Read the model definition and answer for the solid it produces. Units are mm, in the model's axes. Face numbers are marked on the shaded views. Coordinates: 2 decimals unless noted, no trailing zeros. Write each loop counter-clockwise with the first axis right and the second up, starting at its lowest first coordinate (ties: lowest second). Pieces come first, ordered by that corner, then holes.
1) The part is cut by section B-B (y = 0). Determine the outline of the cut face in (x, z).
2) The part is cut by section A-A (x = -6.35). Determine the outline of the cut face in (y, z), then the cut area to 3 significant figures.
3) Find the intervals of material crossed by line 1 (Y direction, x = -4, z = 19); line 2 (Z direction, x = -3.5, y = 1); line 3 (Y direction, x = -6, z = 26), in increasing order.
4) Determine the mould class of the marked faces 1, 2, 3 and 4 for opening direction Y: +Y half, -Y half, draft (parallel to the pull), parting line (faces both ways), or undercut.
5) Each of these flat-tipped pins is pushed along its axis until it touches: pin 1 Ø6 at (y, z) = (-4.5, -7.5) entering from -X; pin 2 Ø12 at (x, z) = (-16, -2) entering from -Y; pin 3 Ø7.5 at (x, y) = (-6.5, 0) entering from +Z. Where does it stop, or does it pass through?
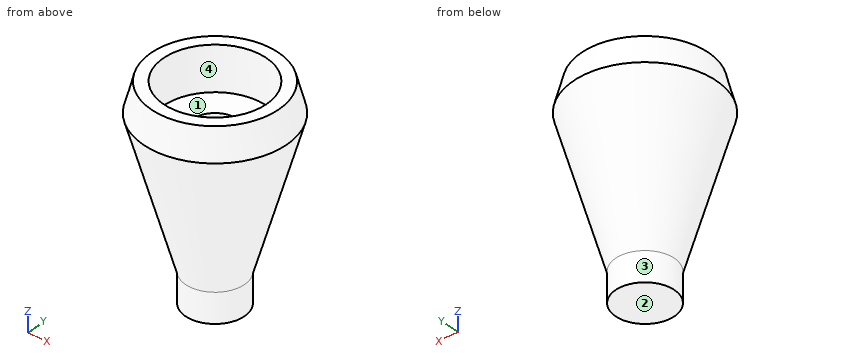
from build123d import *

# Parameters (mm, degrees)
F2_R     = 11.1125
F2_R_2   = 4.7625
F3_DEPTH = 9.525
F4_DEPTH = 31.75


with BuildPart() as f1:
    # F0 (on Front) → F1 (revolve)
    with BuildSketch(Plane.XZ):
        Polygon((-6.35, 29.4268268501), (-6.35, -15.0231731499), (0, -15.0231731499), (0, -8.6731731499), (9.0779721894, 23.0768268501), (7.3764948174, 29.4268268501), align=None)
    revolve(axis=Axis((-6.35, 0, 7.2018268501), (0, 0, -1)))

    # F2 (on face) → F3 (cut)
    with BuildSketch(Plane.XY.offset(29.4268268501)):
        with Locations((-6.35, 0)):
            Circle(F2_R)
        with Locations((-6.35, 0)):
            Circle(F2_R_2, mode=Mode.SUBTRACT)
    extrude(amount=-F3_DEPTH, mode=Mode.SUBTRACT)

    # F4 (cut): a face of the model
    f4_faces = [f1.faces().sort_by_distance(p)[0] for p in [
        (-6.35, 0, 29.4268268501),
    ]]
    extrude(f4_faces, amount=-F4_DEPTH, mode=Mode.SUBTRACT)


solid = f1.part
Reported:
1. outline: (-21.78, 23.08) - (-12.7, -8.67) - (-12.7, -15.02) - (0, -15.02) - (0, -8.67) - (9.08, 23.08) - (7.38, 29.43) - (4.76, 29.43) - (4.76, 19.9) - (-1.59, 19.9) - (-1.59, -2.32) - (-11.11, -2.32) - (-11.11, 19.9) - (-17.46, 19.9) - (-17.46, 29.43) - (-20.08, 29.43) - close
2. outline: (-15.43, 23.08) - (-6.35, -8.67) - (-6.35, -15.02) - (6.35, -15.02) - (6.35, -8.67) - (15.43, 23.08) - (13.73, 29.43) - (11.11, 29.43) - (11.11, 19.9) - (4.76, 19.9) - (4.76, -2.32) - (-4.76, -2.32) - (-4.76, 19.9) - (-11.11, 19.9) - (-11.11, 29.43) - (-13.73, 29.43) - close
2. area: 534 mm2
3. line 1: y = -14.07 to -4.14, 4.14 to 14.07
3. line 2: z = -15.02 to -2.32
3. line 3: y = -14.64 to -11.11, 11.11 to 14.64
4. face 1: undercut
4. face 2: draft
4. face 3: parting line
4. face 4: undercut
5. pin 1: stops at x = -13.25
5. pin 2: stops at y = -7.95
5. pin 3: stops at z = -2.32
